Geometry: final body of the model. Coordinates: model frame, mm. A direction names the side the tool comes from. Round coordinates to 2 decimals unless told otherwise and drop trailing zeros. Loops run counter-clockwise (first coordinate to the right, second up) from the corner with the lowest first, then second, coordinate; pieces in that order, holes last. Notation, with made-up numbers: M 40,-12.75 L 89,-12.75 A25 ccw 89,24.25 Z; hole C 78,77.25 d7. An arc over 180 degrees is marked long. Return JSON: item names as keys, results as strings.
Autodesk Inventor part; units mm, degrees
ref_plane "YZ Plane" through (0, 0, 0) normal (1, 0, 0) x (0, 1, 0)
ref_plane "XZ Plane" through (0, 0, 0) normal (0, 1, 0) x (-1, 0, 0)
ref_plane "XY Plane" through (0, 0, 0) normal (0, 0, 1) x (1, 0, 0)
sketch "Sketch1" plane through (0, 0, 0) normal (0, 0, 1) x (1, 0, 0)
  line L0 (0, 0) -> (50.8, 0)
  line L1 (50.8, 0) -> (50.8, 177.8)
  line L2 (50.8, 177.8) -> (0, 177.8)
  line L3 (0, 177.8) -> (0, 0)
  dimension "d0" = 50.8
  dimension "d1" = 177.8
extrude "Extrusion1" add sketch "Sketch1" along normal blind 25.4
sketch "Sketch2" plane through (0, 177.8, 0) normal (0, 1, 0) x (1, 0, 0)
  line L0 (0, 0) -> (0, -25.4)
  line L1 (50.8, -25.4) -> (0, -25.4)
  line L2 (50.8, 0) -> (50.8, -25.4)
  line L3 (50.8, 0) -> (0, 0)
  line L4 (48.895, -23.495) -> (1.905, -23.495)
  line L5 (1.905, -23.495) -> (1.905, -1.905)
  line L6 (1.905, -1.905) -> (48.895, -1.905)
  line L7 (48.895, -1.905) -> (48.895, -23.495)
  dimension "d4" = 1.905
extrude "Extrusion2" cut sketch "Sketch2" against normal blind 508 contours L4 L5 L6 L7
sketch "Sketch3" plane through (0, 0, 25.4) normal (0, 0, 1) x (1, 0, 0)
  line L0 (1.905, 0) -> (48.895, 0) construction
  line L1 (25.4, 0) -> (25.4, 12.7) construction
  line L2 (25.4, 12.7) -> (25.4, 38.1) construction
  line L3 (48.895, 177.8) -> (1.905, 177.8) construction
  line L4 (25.4, 177.8) -> (25.4, 152.4) construction
  circle A0 centre (25.4, 152.4) radius 14.2557
  circle A1 centre (25.4, 12.7) radius 2.5797
  circle A2 centre (25.4, 38.1) radius 2.5797
  point P0 (0, 0)
  dimension "d7" = 12.7
  dimension "d8" = 25.4
  dimension "d9" = 25.4
  dimension "d10" = 28.5115
  dimension "d11" = 5.1594
  dimension "d12" = 5.1594
extrude "Extrusion3" cut sketch "Sketch3" against normal blind 508
properties part number "vertical leg"
Q1. Section query D-D (y = 103). Output: boundary loops of the cut face in (x, z) (3 decimals), plus the area to 3 significant figures.
Determined:
{"outline": "M 0,0 L 50.8,0 L 50.8,25.4 L 0,25.4 Z; hole M 1.905,1.905 L 48.895,1.905 L 48.895,23.495 L 1.905,23.495 Z", "area": "276 mm^2"}
Q2. Reachability of faces 5 (the flat face through (26, 90, 23.495)), 6 (the flat face through (25, 90, 25.4)) from +Z, -Z, +X, -X, +Y, -Y: full face, straight path, thin tool, end or side. Return the list, or none.
Determined:
{"face 5": "+Y, -Y", "face 6": "+Z, +X, -X, +Y, -Y"}
Q3. Section query C-C (x = 25.4). State how many separate pieces and enclosed holes the cut face has, plus the area to 3 significant figures.
Determined:
{"separate pieces": "8", "enclosed holes": "0", "area": "529 mm^2"}
Q4. Material intervals for L1, parallel to Y at x = 25.4, z = 1.25; L2, parallel to Z at x = 17, y = 52 (3 decimals); L3, parallel to X at y = 102, z = 17 (3 decimals), sorted ascending.
Determined:
{"L1": "y = 0 to 10.12, 15.28 to 35.52, 40.68 to 138.14, 166.66 to 177.8", "L2": "z = 0 to 1.905, 23.495 to 25.4", "L3": "x = 0 to 1.905, 48.895 to 50.8"}
Q5. Section query B-B (z = 5.25). Output: boundary loops of the cut face in (x, y) (3 decimals).
Determined:
{"outline": "M 0,0 L 1.905,0 L 1.905,177.8 L 0,177.8 Z; M 48.895,0 L 50.8,0 L 50.8,177.8 L 48.895,177.8 Z"}
Q6. Section query A-A (y = 12.7). Output: boundary loops of the cut face in (x, z) (3 decimals).
Determined:
{"outline": "M 0,0 L 22.82,0 L 22.82,1.905 L 1.905,1.905 L 1.905,23.495 L 22.82,23.495 L 22.82,25.4 L 0,25.4 Z; M 27.98,0 L 50.8,0 L 50.8,25.4 L 27.98,25.4 L 27.98,23.495 L 48.895,23.495 L 48.895,1.905 L 27.98,1.905 Z"}
Q7. Pull-direction query (Y, two-part tool) for faces 1 (the flat face through (48.895, 90, 13)), 2 (the cylindrical face through (26.59, 35.81, 0.97)), 3 (the cylindrical face through (27.783, 11.712, 0.966)), 4 (the flat face through (27, 177.8, 24)); classes: pulls with the +Y half, pulls with the -Y half, needs draft (parallel to the pull), parting line crosses it, or undercut.
Determined:
{"face 1": "needs draft", "face 2": "undercut", "face 3": "undercut", "face 4": "pulls with the +Y half"}
